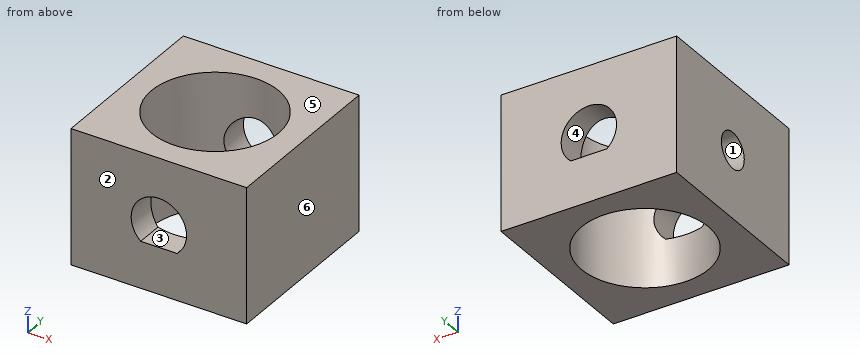
from build123d import *

# Parameters (mm, degrees)
SKETCH1_W           = 13
SKETCH1_H           = 10
BOSS_EXTRUDE1_DEPTH = 13
SKETCH2_R           = 4.7
CUT_EXTRUDE1_DEPTH  = 10
CUT_EXTRUDE2_REACH  = 15
SKETCH3_R           = 1.325


with BuildPart() as part:
    # Sketch1 → Boss-Extrude1 (new body)
    with BuildSketch(Plane(origin=(0, 0, 0), x_dir=(1, 0, 0), z_dir=(0, 1, 0))):
        Rectangle(SKETCH1_W, SKETCH1_H)
        with BuildLine():
            Line((-1.341640786, 1.55), (1.341640786, 1.55))
            ThreePointArc((1.341640786, 1.55), (0, -2.05), (-1.341640786, 1.55))
        make_face(mode=Mode.SUBTRACT)
    extrude(amount=BOSS_EXTRUDE1_DEPTH)

    # Sketch2 → Cut-Extrude1 (cut)
    with BuildSketch(Plane.XY.offset(5)):
        with Locations((0, 6.5)):
            Circle(SKETCH2_R)
    extrude(amount=-CUT_EXTRUDE1_DEPTH, mode=Mode.SUBTRACT)

    # Sketch3 → Cut-Extrude2 (cut, up to next)
    with BuildSketch(Plane.ZY.offset(6.5), mode=Mode.PRIVATE) as cut_extrude2_sk1:
        with Locations((0, 6.5)):
            Circle(SKETCH3_R)
    cut_extrude2_tool1 = extrude(cut_extrude2_sk1.sketch, amount=-CUT_EXTRUDE2_REACH, mode=Mode.PRIVATE) & part.part
    add(cut_extrude2_tool1.solids().sort_by_distance((-6.5, 6.5, 0))[0], mode=Mode.SUBTRACT)


solid = part.part
CAD build for the part. Positions are in the model's coordinates, mm. Face numbers are marked on the shaded views. A direction names the side the tool comes from. Give positions to 0.01 mm unless a question says otherwise; leave off trailing zeros. Loops run counter-clockwise (first coordinate to the right, second up) from the corner with the lowest first, then second, coordinate; pieces in that order, holes last. Notation, with made-up numbers: M 12,3 L 47,3 A33 cw 47,41 Z; hole C 79.25,-26.5 d2. An arc over 180 degrees is marked long. Answer in a Markdown table with one row per item. Add a question column.
Item 1: Probe probe 1 along X at (y, z) = (6.5, 1.75); probe 2 along Z at (x, y) = (-5, 6.5) (3 decimals); probe 3 along X at (y, z) = (1.7, 0). List the from-to ranges inside material, lowest first.
Item 2: Mould opens along X. For the marked faces 4, 5 and 6 say: +X half, -X half, draft (parallel to the pull), parting line (faces both ways), or undercut.
Item 3: Drop a flat-ended pin along its axis: P1, Ø2.5, axis at x = 0, z = 0, coming from the -Y side. Give the stop position or say it passes through.
Item 4: Band-saw the part on B-B on y = 11.5. Give the cut face in (x, z), then the cut area to 3 significant figures.
Item 5: Band-saw the part on D-D on y = 6.5. Give the cut face in (x, z) (3 decimals), then the cut area to 3 significant figures.
Item 6: Band-saw the part on A-A on x = 0. Give the cut face in (y, z).
Item 7: Tool access for the marked faces 1, 2 and 3: list every direction of +Z, -Z, +X, -X, +Y, -Y with a clear straight run to the whole face (end or side of a thin tool).
Item 8: Band-saw the part on C-C on z = 0.25. Give the cut face in (x, y).
Reply:
| question | item | result |
|---|---|---|
| 1 | probe 1 | x = -6.5 to -4.7, 4.7 to 6.5 |
| 1 | probe 2 | z = -5 to -1.325, 1.325 to 5 |
| 1 | probe 3 | x = -6.5 to -2.05, 2.05 to 6.5 |
| 2 | face 4 | undercut |
| 2 | face 5 | draft |
| 2 | face 6 | +X half |
| 3 | P1 | passes through |
| 4 | outline | M -6.5,-5 L 6.5,-5 L 6.5,5 L -6.5,5 Z; hole M -1.34,-1.55 L 1.34,-1.55 A2.05 ccw long Z |
| 4 | area | 118 mm^2 |
| 5 | outline | M -6.5,-5 L -4.7,-5 L -4.7,-1.325 L -6.5,-1.325 Z; M -6.5,1.325 L -4.7,1.325 L -4.7,5 L -6.5,5 Z; M 4.7,-5 L 6.5,-5 L 6.5,5 L 4.7,5 Z |
| 5 | area | 31.2 mm^2 |
| 6 | outline | M 0,-5 L 1.8,-5 L 1.8,-1.55 L 0,-1.55 Z; M 0,2.05 L 1.8,2.05 L 1.8,5 L 0,5 Z; M 11.2,-5 L 13,-5 L 13,-1.55 L 11.2,-1.55 Z; M 11.2,2.05 L 13,2.05 L 13,5 L 11.2,5 Z |
| 7 | face 1 | -X |
| 7 | face 2 | +Z, -Z, +X, -X, -Y |
| 7 | face 3 | +Y, -Y |
| 8 | outline | M -6.5,0 L -2.03,0 L -2.03,2.26 A4.7 cw -4.52,5.2 L -6.5,5.2 Z; M -6.5,7.8 L -4.52,7.8 A4.7 cw -2.03,10.74 L -2.03,13 L -6.5,13 Z; M 2.03,0 L 6.5,0 L 6.5,13 L 2.03,13 L 2.03,10.74 A4.7 cw 2.03,2.26 Z |
